```python
from build123d import *

# Parameters (mm, degrees)
F0_W     = 54
F0_H     = 28
F1_DEPTH = 4


# Not quite as in the source:
# - a feature of the source that left no trace in its solid (it failed there, or was rolled back) is left out


with BuildPart() as f1:
    # F0 (on Top) → F1 (new body)
    with BuildSketch(Plane.XY):
        with BuildLine():
            Line((14, -45), (14, -53.1883445879))
            ThreePointArc((14, -53.1883445879), (21.0475887801, -50.8133742881), (27.7103442016, -47.5093340748))
            Line((27.7103442016, -47.5093340748), (21.9203102168, -41.71930009))
            Line((21.9203102168, -41.71930009), (41.71930009, -21.9203102168))
            Line((41.71930009, -21.9203102168), (47.5093340748, -27.7103442016))
            ThreePointArc((47.5093340748, -27.7103442016), (50.8133742881, -21.0475887801), (53.1883445879, -14))
            Line((53.1883445879, -14), (45, -14))
            Line((45, -14), (45, 14))
            Line((45, 14), (53.1883445879, 14))
            ThreePointArc((53.1883445879, 14), (50.8133742881, 21.0475887801), (47.5093340748, 27.7103442016))
            Line((47.5093340748, 27.7103442016), (41.0177921349, 21.2188022616))
            Line((41.0177921349, 21.2188022616), (21.2188022616, 41.0177921349))
            Line((21.2188022616, 41.0177921349), (27.7103442016, 47.5093340748))
            ThreePointArc((27.7103442016, 47.5093340748), (21.0475887801, 50.8133742881), (14, 53.1883445879))
            Line((14, 53.1883445879), (14, 45))
            Line((14, 45), (-14, 45))
            Line((-14, 45), (-14, 53.1883445879))
            ThreePointArc((-14, 53.1883445879), (-21.0475887801, 50.8133742881), (-27.7103442016, 47.5093340748))
            Line((-27.7103442016, 47.5093340748), (-21.9203102168, 41.71930009))
            Line((-21.9203102168, 41.71930009), (-41.71930009, 21.9203102168))
            Line((-41.71930009, 21.9203102168), (-47.5093340748, 27.7103442016))
            ThreePointArc((-47.5093340748, 27.7103442016), (-50.8133742881, 21.0475887801), (-53.1883445879, 14))
            Line((-53.1883445879, 14), (-45, 14))
            Line((-45, 14), (-45, -14))
            Line((-45, -14), (-53.1883445879, -14))
            ThreePointArc((-53.1883445879, -14), (-50.8133742881, -21.0475887801), (-47.5093340748, -27.7103442016))
            Line((-47.5093340748, -27.7103442016), (-41.71930009, -21.9203102168))
            Line((-41.71930009, -21.9203102168), (-21.9203102168, -41.71930009))
            Line((-21.9203102168, -41.71930009), (-27.7103442016, -47.5093340748))
            ThreePointArc((-27.7103442016, -47.5093340748), (-21.0475887801, -50.8133742881), (-14, -53.1883445879))
            Line((-14, -53.1883445879), (-14, -45))
            Line((-14, -45), (14, -45))
        make_face()
        Rectangle(F0_W, F0_H, mode=Mode.SUBTRACT)
    extrude(amount=F1_DEPTH)


solid = f1.part
```
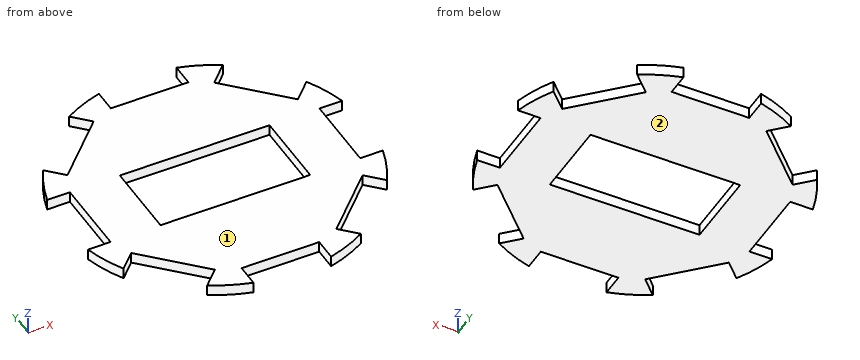
For this review, take the finished solid that the model builds, in its own axes (mm). Face numbers are marked on the shaded views. Round coordinates to 2 decimals unless told otherwise and drop trailing zeros. Order: outer loops, then holes, each group sorted by start corner. A loop starts at its lowest first (then second) coordinate and runs counter-clockwise, first axis right, second up.
Q1. We need section D-D, the plane x = 30. Give the boundary of the cut face in (y, z), plus the area to 3 significant figures.
Findings below:
outline: (-33.64, 0) - (32.24, 0) - (32.24, 4) - (-33.64, 4) - close
area: 264 mm2
Q2. Mouldability with a two-part tool opening along Z and no side actions: class the marked faces 1 and 2 as pulls with the +Z half, pulls with the -Z half, needs draft (parallel to the pull), parting line crosses it, or undercut.
Findings below:
face 1: pulls with the +Z half
face 2: pulls with the -Z half
Q3. We need section B-B, the plane y = -8.5. Give the boundary of the cut face in (x, z), plus the area to 3 significant figures.
Findings below:
outline: (-45, 0) - (-27, 0) - (-27, 4) - (-45, 4) - close; (27, 0) - (45, 0) - (45, 4) - (27, 4) - close
area: 144 mm2
Q4. We need section A-A, the plane x = 4. Give the boundary of the cut face in (y, z).
Findings below:
outline: (-45, 0) - (-14, 0) - (-14, 4) - (-45, 4) - close; (14, 0) - (45, 0) - (45, 4) - (14, 4) - close
Q5. Wall thickness on line 1 (X direction, y = 25.5, z = 3.1); line 2 (Y direction, x = -23, z = 1.6); line 3 (Y direction, x = -11, z = 2.15): over which ranges is each line inside the solid? List them lowest first.
Findings below:
line 1: x = -48.73 to -45.3, -38.14 to 36.74, 45.3 to 48.73
line 2: y = -49.96 to -42.8, -40.64 to -14, 14 to 40.64, 42.8 to 49.96
line 3: y = -45 to -14, 14 to 45
Q6. Insertion check: P1, Ø1.5, axis at x = -28, z = 0.5, coming from the +Y side; P2, Ø1.5, axis at y = 31, z = 1, coming from the +X side; P3, Ø4, axis at x = -25.5, y = -14.5, coming from the -Z side; P4, Ø1.2, axis at x = -48.5, z = 1.5, coming from the -Y side. Each pin has a flat end and moves straight along its axis. Give the tip position at first contact, or say it passes through.
Findings below:
P1: stops at y = 47.77
P2: stops at x = 31.99
P3: stops at z = 0
P4: stops at y = -27.03
Q7. We need section C-C, the plane y = 23.5. Give the boundary of the cut face in (x, z), plus the area to 3 significant figures.
Findings below:
outline: (-49.73, 0) - (-43.3, 0) - (-43.3, 4) - (-49.73, 4) - close; (-40.14, 0) - (38.74, 0) - (38.74, 4) - (-40.14, 4) - close; (43.3, 0) - (49.73, 0) - (49.73, 4) - (43.3, 4) - close
area: 367 mm2
